Source: three-view drawing plus pictorial views. Frame: mm from the lowest corner of the part. A direction names the side the tool comes from. Give positions to 0.01 mm unless a question says otherwise; leave off trailing zeros. Write each loop counter-clockwise with the first axis right and the second up, starting at its lowest first coordinate (ties: lowest second). Pieces come first, ordered by that corner, then holes. Notation, with made-up numbers: M 56.25,68 L 110.25,68 A7 cw 110.25,73 Z; hole C -32.5,46 d9. An arc over 180 degrees is marked long. Return JSON: item names as keys, results as strings.
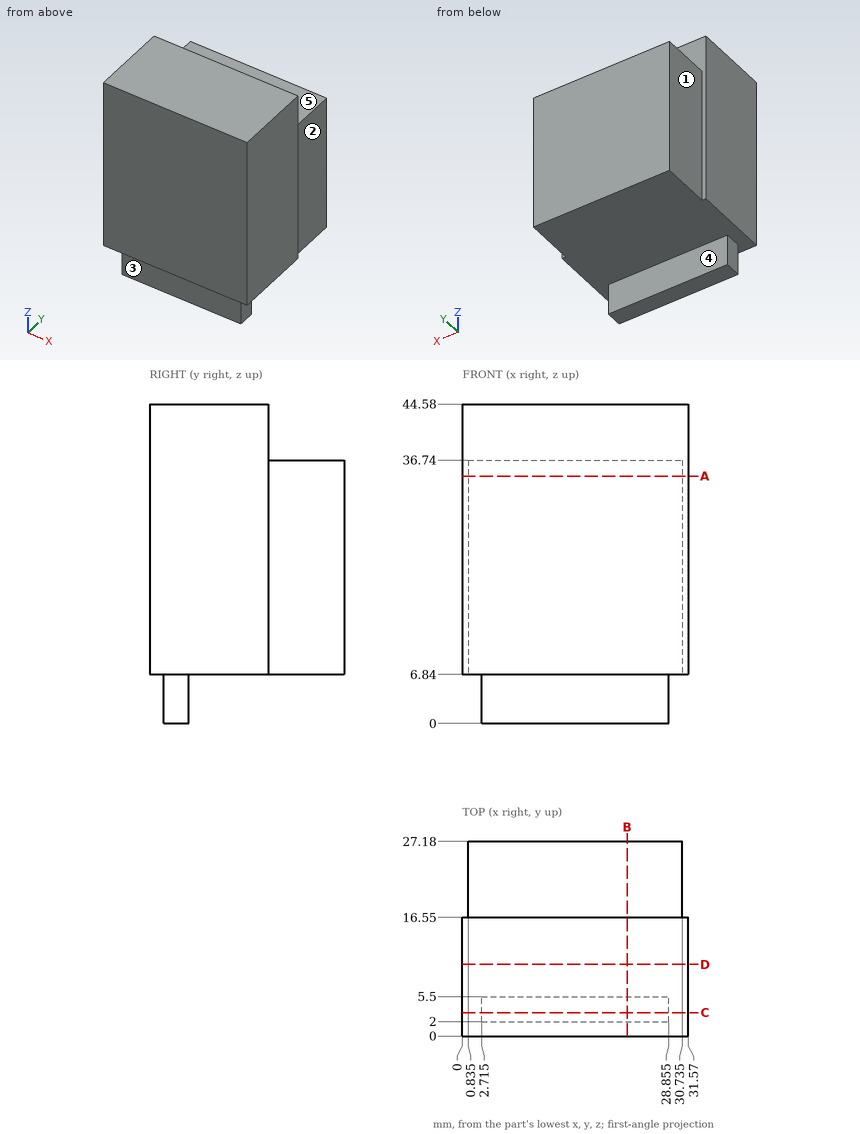
1) Cut plane D-D, the plane y = 10. Return the cut outline in (x, z).
Numbers:
{"outline": "M 0,6.84 L 31.57,6.84 L 31.57,44.58 L 0,44.58 Z"}
2) Contact query for flat-ended pins moving along their axis: pin 1 Ø3 at (y, z) = (24, 27) entering from +X (3 decimals); pin 2 Ø3 at (y, z) = (3, 3) entering from +X (3 decimals); pin 3 Ø4 at (y, z) = (13, 19.5) entering from -X; pin 4 Ø2 at (x, z) = (13.5, 4) entering from -Y. Output: stop coordinate, or through.
Numbers:
{"pin 1": "stops at x = 30.735", "pin 2": "stops at x = 28.855", "pin 3": "stops at x = 0", "pin 4": "stops at y = 2"}
3) Set-up query: the marked faces 1, 2, 3, 4 and 5. Return all of +Z, -Z, +X, -X, +Y, -Y with unobstructed straight access to the full face (end or side cutting, diameter ignored); none if empty.
Numbers:
{"face 1": "+Z, -Z, -X, +Y", "face 2": "+Z, -Z, +X, +Y", "face 3": "-Z, +X, -X, -Y", "face 4": "-Z, +X, -X, +Y", "face 5": "+Z, +X, -X, +Y"}
4) Cut plane C-C, the plane y = 3.25. Return the cut outline in (x, z) (3 decimals).
Numbers:
{"outline": "M 0,6.84 L 2.715,6.84 L 2.715,0 L 28.855,0 L 28.855,6.84 L 31.57,6.84 L 31.57,44.58 L 0,44.58 Z"}
5) Cut plane B-B, the plane x = 23. Return the cut outline in (y, z), then the cut area to 3 significant figures.
Numbers:
{"outline": "M 0,6.84 L 2,6.84 L 2,0 L 5.5,0 L 5.5,6.84 L 27.18,6.84 L 27.18,36.74 L 16.55,36.74 L 16.55,44.58 L 0,44.58 Z", "area": "966 mm²"}
6) Cut plane A-A, the plane z = 34.5. Return the cut outline in (x, y) (3 decimals), then the cut area to 3 significant figures.
Numbers:
{"outline": "M 0,0 L 31.57,0 L 31.57,16.55 L 30.735,16.55 L 30.735,27.18 L 0.835,27.18 L 0.835,16.55 L 0,16.55 Z", "area": "840 mm²"}
7) Line query: line 1 (Z direction, x = 7, y = 1.5); line 2 (Z direction, x = 25, y = 20.75); line 3 (Y direction, x = 8.5, z = 39). Output: solid intervals per line, ascending. Write a range as [from, to].
Numbers:
{"line 1": "z = [6.84, 44.58]", "line 2": "z = [6.84, 36.74]", "line 3": "y = [0, 16.55]"}
